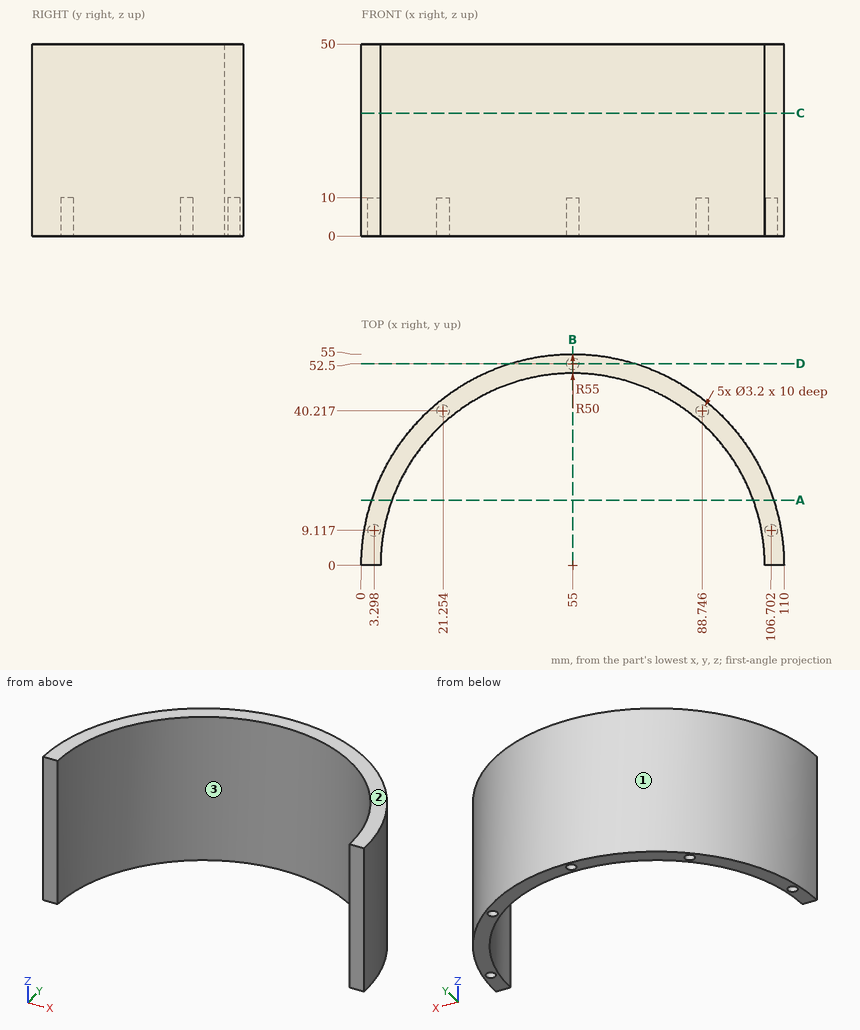
Geometry: see drawing. Coordinates: mm, zero at the bounding-box minimum. Coordinates: 2 decimals unless noted, no trailing zeros. Loops run counter-clockwise (first coordinate to the right, second up) from the corner with the lowest first, then second, coordinate; pieces in that order, holes last.
(1) First-contact query: pin 1 Ø1 at (x, y) = (54.5, 53) entering from -Z; pin 2 Ø2 at (x, z) = (90, 28.5) entering from -Y; pin 3 Ø4 at (y, z) = (20, 35.5) entering from -X; pin 4 Ø2.5 at (x, y) = (3, 8.5) entering from -Z. Flat tips, straight axial feed; report the tip coordinate or a pass-through.
(2) Section C-C on z = 32. Return the cut outline in (x, y).
(3) Section B-B on x = 55. Return the cut outline in (y, z), then the cut area to 3 significant figures.
(4) Pull-direction query (X, two-part tool) for the marked faces 1, 2 and 3; classes: released by +X, released by -X, zero draft, split by the parting line, or undercut.
(5) Material intervals for probe 1 along X at (y, z) = (34.5, 17.5) (1 decimal); probe 2 along X at (y, z) = (40, 16); probe 3 along Y at (x, z) = (92.5, 7) (1 decimal), sorted ascending.
(6) Section A-A on y = 17. Return the cut outline in (x, z).
(7) Section D-D on y = 52.5. Return the cut outline in (x, z), then the cut area to 3 significant figures.
Data:
1. pin 1: stops at z = 10
1. pin 2: stops at y = 34.7
1. pin 3: stops at x = 3.03
1. pin 4: stops at z = 0
2. outline: (0, 0) - (5, 0) arc R50 cw to (105, 0) - (110, 0) arc R55 ccw to start
3. outline: (50, 0) - (50.9, 0) - (50.9, 10) - (54.1, 10) - (54.1, 0) - (55, 0) - (55, 50) - (50, 50) - close
3. area: 218 mm2
4. face 1: split by the parting line
4. face 2: zero draft
4. face 3: undercut
5. probe 1: x = 12.2 to 18.8, 91.2 to 97.8
5. probe 2: x = 17.25 to 25, 85 to 92.75
5. probe 3: y = 33.1 to 40.2
6. outline: (2.69, 0) - (7.98, 0) - (7.98, 50) - (2.69, 50) - close; (102.02, 0) - (107.31, 0) - (107.31, 50) - (102.02, 50) - close
7. outline: (38.61, 0) - (53.4, 0) - (53.4, 10) - (56.6, 10) - (56.6, 0) - (71.39, 0) - (71.39, 50) - (38.61, 50) - close
7. area: 1,610 mm2
